Verification items for the finished model (mm, model axes). Face numbers are marked on the shaded views. Coordinates: 2 decimals unless noted, no trailing zeros. Order: outer loops, then holes, each group sorted by start corner. A loop starts at its lowest first (then second) coordinate and runs counter-clockwise, first axis right, second up. Notation, with made-up numbers: (-27, 60) -> (6, 60) arc R12 cw to (6, 71) -> close; hole circle Ø2 at (33, 75). An arc over 180 degrees is marked (long way). Write item = value, one per line. Start each with the question number.
1. Cross-section at A-A on x = 0. Record the cut outline in (y, z) (3 decimals).
2. Release check for a two-part mould opening along X. For the marked faces 1, 2 and 3 record: +X half, -X half, draft (parallel to the pull), parting line (faces both ways), or undercut.
3. Thickness scan on line 1 along Y through (x, z) = (0, 9.5) (3 decimals); line 2 along Z through (x, y) = (0.15, 1.2); line 3 along X through (y, z) = (1.35, 5). Record the ranges inside material, lowest first. Write a range as from..to.
4. Cross-section at C-C on z = 15. Record the cut outline in (x, y) (3 decimals), plus the area to 3 significant figures.
5. Go/stop test with flat-tipped pins: P1, Ø1.5, axis at y = 1.5, z = 4.5, coming from the +X side; P2, Ø1, axis at x = 1.5, z = 13, coming from the -Y side; P3, Ø1.2, axis at x = 0, y = 0, coming from the +Z side. Record where each tip stops, or that it passes through.
6. Cross-section at B-B on z = 6.25. Record the cut outline in (x, y) (3 decimals).
from build123d import *

# Parameters (mm, degrees)
SKETCH1_R           = 2.775
BOSS_EXTRUDE1_DEPTH = 18
SKETCH2_R           = 2.27
CUT_EXTRUDE1_DEPTH  = 5.68
CUT_EXTRUDE1_TAPER  = 3.074
SKETCH7_R           = 1
CUT_EXTRUDE2_DEPTH  = 19
SKETCH9_R           = 2.27
CUT_EXTRUDE3_DEPTH  = 5.68
CUT_EXTRUDE3_TAPER  = 3.074


with BuildPart() as part:
    # Sketch1 → Boss-Extrude1 (new body)
    with BuildSketch(Plane.XY):
        Circle(SKETCH1_R)
    extrude(amount=BOSS_EXTRUDE1_DEPTH)

    # Sketch2 → Cut-Extrude1 (cut)
    with BuildSketch(Plane.XY):
        Circle(SKETCH2_R)
    extrude(amount=CUT_EXTRUDE1_DEPTH, taper=CUT_EXTRUDE1_TAPER, mode=Mode.SUBTRACT)

    # Sketch7 → Cut-Extrude2 (cut, through all)
    with BuildSketch(Plane.XY):
        Circle(SKETCH7_R)
    extrude(amount=CUT_EXTRUDE2_DEPTH, mode=Mode.SUBTRACT)

    # Sketch9 → Cut-Extrude3 (cut)
    with BuildSketch(Plane.XY.offset(18)):
        Circle(SKETCH9_R)
    extrude(amount=-CUT_EXTRUDE3_DEPTH, taper=CUT_EXTRUDE3_TAPER, mode=Mode.SUBTRACT)


solid = part.part
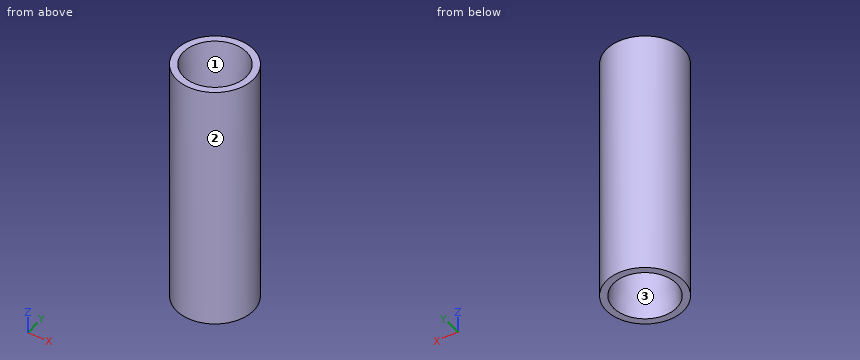
Worked out:
q1.outline = (-2.775, 0) -> (-2.27, 0) -> (-1.965, 5.68) -> (-1, 5.68) -> (-1, 12.32) -> (-1.965, 12.32) -> (-2.27, 18) -> (-2.775, 18) -> close; (1, 5.68) -> (1.965, 5.68) -> (2.27, 0) -> (2.775, 0) -> (2.775, 18) -> (2.27, 18) -> (1.965, 12.32) -> (1, 12.32) -> close
q2.face_1 = undercut
q2.face_2 = parting line
q2.face_3 = undercut
q3.line_1 = -2.775..-1, 1..2.775
q3.line_2 = 5.68..12.32
q3.line_3 = -2.42..-1.48, 1.48..2.42
q4.outline = circle Ø5.55 at (0, 0); hole circle Ø4.218 at (0, 0)
q4.area = 10.2 mm²
q5.P1 = 2.67
q5.P2 = -2.59
q5.P3 = through
q6.outline = circle Ø5.55 at (0, 0); hole circle Ø2 at (0, 0)
